Geometry check sheet. Reference: the model listing, model coordinates, mm. A direction names the side the tool comes from. Coordinates: 2 decimals unless noted, no trailing zeros. Write each loop counter-clockwise with the first axis right and the second up, starting at its lowest first coordinate (ties: lowest second). Pieces come first, ordered by that corner, then holes. Notation, with made-up numbers: M -1.5,52 L 53.5,52 A27 ccw 53.5,87 Z; hole C 32.5,42.5 d5. An arc over 180 degrees is marked long. Write each question's results on one line, items separated by ' | '.
```python
from build123d import *

# Parameters (mm, degrees)
BOSS_EXTRUDE1_DEPTH             = 25.4
SKETCH2_R                       = 3.81
CUT_EXTRUDE1_DEPTH              = 95.74063806
F_1_4_0_25_DIAMETER_HOLE1_D     = 6.35
F_1_4_0_25_DIAMETER_HOLE1_DEPTH = 7.62
F_1_4_0_25_DIAMETER_HOLE1_TIP   = 1.907732465
F_1_4_0_25_DIAMETER_HOLE2_D     = 6.35
F_1_4_0_25_DIAMETER_HOLE2_DEPTH = 10.16
F_1_4_0_25_DIAMETER_HOLE2_TIP   = 1.907732465


with BuildPart() as part:
    # Sketch1 → Boss-Extrude1 (new body)
    with BuildSketch(Plane(origin=(0, 0, 0), x_dir=(1, 0, 0), z_dir=(0, 1, 0))):
        Polygon((69.85, 0), (85.09, 0), (85.09, 5.08), (73.66, 5.08), (73.66, 15.24), (85.09, 15.24), (85.09, 33.02), (0, 33.02), (0, 15.24), (11.43, 15.24), (11.43, 5.08), (0, 5.08), (0, 0), (15.24, 0), (15.24, 27.94), (69.85, 27.94), align=None)
    extrude(amount=BOSS_EXTRUDE1_DEPTH)

    # Sketch2 → Cut-Extrude1 (cut, through all)
    with BuildSketch(Plane(origin=(0, 25.4, 0), x_dir=(1, 0, 0), z_dir=(0, 1, 0))):
        with Locations(Location((7.62, 22.86, 0), (0, 0, 270))):
            Circle(SKETCH2_R)
        with Locations(Location((77.47, 22.86, 0), (0, 0, 270))):
            Circle(SKETCH2_R)
    extrude(amount=-CUT_EXTRUDE1_DEPTH, mode=Mode.SUBTRACT)

    # 1/4 (0.25) Diameter Hole1
    with Locations(Plane.XY):
        with Locations((5.715, 13.802822473), (79.375, 13.802822473)):
            Hole(F_1_4_0_25_DIAMETER_HOLE1_D / 2, depth=F_1_4_0_25_DIAMETER_HOLE1_DEPTH)
            with Locations((0, 0, -(F_1_4_0_25_DIAMETER_HOLE1_DEPTH + F_1_4_0_25_DIAMETER_HOLE1_TIP / 2))):  # 118° drill point
                Cone(0, F_1_4_0_25_DIAMETER_HOLE1_D / 2, F_1_4_0_25_DIAMETER_HOLE1_TIP, mode=Mode.SUBTRACT)

    # 1/4 (0.25) Diameter Hole2
    with Locations(Plane(origin=(0, 0, -33.02), x_dir=(-1, 0, 0), z_dir=(0, 0, -1))):
        with Locations((-77.47, 12.7), (-7.62, 12.7)):
            Hole(F_1_4_0_25_DIAMETER_HOLE2_D / 2, depth=F_1_4_0_25_DIAMETER_HOLE2_DEPTH)
            with Locations((0, 0, -(F_1_4_0_25_DIAMETER_HOLE2_DEPTH + F_1_4_0_25_DIAMETER_HOLE2_TIP / 2))):  # 118° drill point
                Cone(0, F_1_4_0_25_DIAMETER_HOLE2_D / 2, F_1_4_0_25_DIAMETER_HOLE2_TIP, mode=Mode.SUBTRACT)


solid = part.part
```
Q1. Scan lines: probe 1 along X at (y, z) = (8.5, -22.86); probe 2 along X at (y, z) = (23.75, -2.5); probe 3 along X at (y, z) = (1.75, -6.5). Record each from-to range of solid material in increasing order.
Geometry check:
probe 1: x = 0 to 3.81, 11.43 to 15.24, 69.85 to 73.66, 81.28 to 85.09 | probe 2: x = 0 to 15.24, 69.85 to 85.09 | probe 3: x = 11.43 to 15.24, 69.85 to 73.66
Q2. Sectioned sample at B-B on y = 19.5. Record the cut outline in (x, z).
Geometry check:
outline: M 0,-33.02 L 85.09,-33.02 L 85.09,-15.24 L 73.66,-15.24 L 73.66,-5.08 L 85.09,-5.08 L 85.09,0 L 69.85,0 L 69.85,-27.94 L 15.24,-27.94 L 15.24,0 L 0,0 L 0,-5.08 L 11.43,-5.08 L 11.43,-15.24 L 0,-15.24 Z; hole C 7.62,-22.86 d7.62; hole C 77.47,-22.86 d7.62
Q3. Mould release check, pull along X, two halves, no side actions. Record for faces 1 (the flat face through (9, 13, 0)), 2 (the cylindrical face through (6.13, 16.95, -2.58)), 3 (the flat face through (85.09, 13, -24)): pulls with the +X half, pulls with the -X half, needs draft (parallel to the pull), parting line crosses it, or undercut.
Geometry check:
face 1: needs draft | face 2: undercut | face 3: pulls with the +X half
Q4. Sectioned sample at A-A on z = -22.86. Record the cut outline in (x, y).
Geometry check:
outline: M 0,0 L 3.81,0 L 3.81,25.4 L 0,25.4 Z; M 11.43,0 L 15.24,0 L 15.24,25.4 L 11.43,25.4 Z; M 69.85,0 L 73.66,0 L 73.66,25.4 L 69.85,25.4 Z; M 81.28,0 L 85.09,0 L 85.09,25.4 L 81.28,25.4 Z
Q5. Sectioned sample at C-C on x = 7.62. Record the cut outline in (y, z) (3 decimals), and give its area (3 significant figures).
Geometry check:
outline: M 0,-33.02 L 9.525,-33.02 L 9.525,-26.67 L 0,-26.67 Z; M 0,-19.05 L 25.4,-19.05 L 25.4,-15.24 L 0,-15.24 Z; M 0,-5.08 L 11.263,-5.08 L 11.263,0 L 0,0 Z; M 15.875,-33.02 L 25.4,-33.02 L 25.4,-26.67 L 15.875,-26.67 Z; M 16.343,-5.08 L 25.4,-5.08 L 25.4,0 L 16.343,0 Z | area: 321 mm2
Q6. Depth check by flat-ended pin: P1, Ø4.5, axis at x = 77.47, z = -22.86, coming from the +Y side; P2, Ø4, axis at x = 7.62, y = 12.7, coming from the -Z side; P3, Ø4, axis at x = 79.38, y = 13.8, coming from the +Z side. Enter the tip coordinate at first touch or a pass-through.
Geometry check:
P1: passes through | P2: stops at z = -19.62 | P3: stops at z = -15.24
Q7. Sectioned sample at D-D on z = -3. Record the cut outline in (x, y) (3 decimals).
Geometry check:
outline: M 0,0 L 15.24,0 L 15.24,25.4 L 0,25.4 Z; M 69.85,0 L 85.09,0 L 85.09,25.4 L 69.85,25.4 Z; hole C 5.715,13.803 d6.35; hole C 79.375,13.803 d6.35
Q8. Access from +Z, -Z, +X, -X, +Y, -Y to the whole of each face (thin tool, end or side, straight path). Record for faces 4 (the cylindrical face through (8.764, 12.878, -19.226)), 5 (the cylindrical face through (80.5, 13.65, -29.83)), 6 (the flat face through (15.24, 13, -14)), 7 (the flat face through (6, 10, -5.08)), 8 (the flat face through (79, 10, -5.08)).
Geometry check:
face 4: +Y, -Y | face 5: -Z | face 6: +Z, +Y, -Y | face 7: -X, +Y, -Y | face 8: +X, +Y, -Y
